For this review, take the finished solid that the model builds, in its own axes (mm). Face numbers are marked on the shaded views. A direction names the side the tool comes from. Give positions to 0.01 mm unless a question says otherwise; leave off trailing zeros. Loops run counter-clockwise (first coordinate to the right, second up) from the corner with the lowest first, then second, coordinate; pieces in that order, holes last.
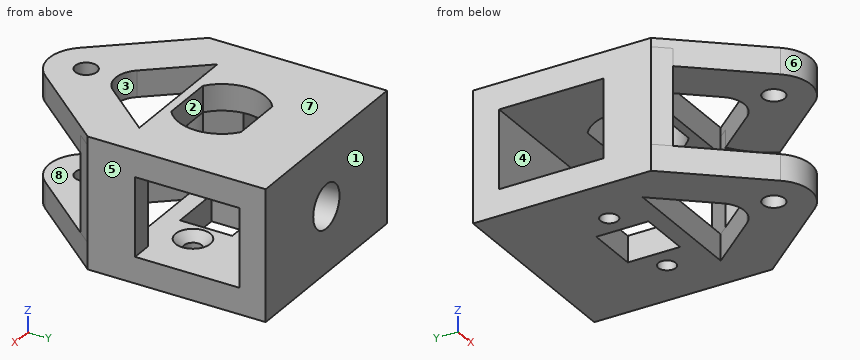
```python
from build123d import *

# Parameters (mm, degrees)
SKETCH1_R           = 1.25
BOSS_EXTRUDE1_DEPTH = 3
BOSS_EXTRUDE2_DEPTH = 14
FILLET1_R           = 1
FILLET3_R           = 3
CUT_EXTRUDE1_DEPTH  = 15
SKETCH8_W           = 23.078375234
SKETCH8_H           = 15
BOSS_EXTRUDE6_DEPTH = 15
SKETCH9_W           = 9
SKETCH9_H           = 12
CUT_EXTRUDE4_DEPTH  = 12.5
SKETCH10_W          = 3
SKETCH10_H          = 2
BOSS_EXTRUDE8_DEPTH = 11.5
CUT_EXTRUDE5_START  = 12
CUT_EXTRUDE5_DEPTH  = 3
SKETCH12_R          = 1
SKETCH12_W          = 6
SKETCH12_H          = 6
CUT_EXTRUDE6_DEPTH  = 3
CUT_EXTRUDE7_START  = 27.589042
SKETCH13_R          = 2.5
CUT_EXTRUDE7_DEPTH  = 4
CHAMFER1_SIZE       = 1


with BuildPart() as part:
    # Sketch1 → Boss-Extrude1 (new body)
    with BuildSketch(Plane.XY):
        with BuildLine():
            Line((-16.111441077, 12.589041521), (-3.255688883, -2.731847341))
            ThreePointArc((-3.255688883, -2.731847341), (0, -4.25), (3.255688883, -2.731847341))
            Line((3.255688883, -2.731847341), (16.111441077, 12.589041521))
            Line((16.111441077, 12.589041521), (9.111441077, 12.589041521))
            Line((9.111441077, 12.589041521), (0, 1.730448884))
            Line((0, 1.730448884), (-9.111441077, 12.589041521))
            Line((-9.111441077, 12.589041521), (-16.111441077, 12.589041521))
        make_face()
        Circle(SKETCH1_R, mode=Mode.SUBTRACT)
    boss_extrude1 = extrude(amount=BOSS_EXTRUDE1_DEPTH)

    # Sketch2 → Boss-Extrude2 (add)
    with BuildSketch(Plane.XY):
        with BuildLine():
            Line((16.111441077, 12.589041521), (9.111441077, 12.589041521))
            Line((9.111441077, 12.589041521), (6.505319132, 9.483186331))
            ThreePointArc((6.505319132, 9.483186331), (8.555448033, 7.684680147), (10.124424164, 5.453992606))
            Line((10.124424164, 5.453992606), (16.111441077, 12.589041521))
        make_face()
        with BuildLine():
            Line((-9.111441077, 12.589041521), (-16.111441077, 12.589041521))
            Line((-16.111441077, 12.589041521), (-10.124424164, 5.453992606))
            ThreePointArc((-10.124424164, 5.453992606), (-8.555448033, 7.684680147), (-6.505319132, 9.483186331))
            Line((-6.505319132, 9.483186331), (-9.111441077, 12.589041521))
        make_face()
    extrude(amount=BOSS_EXTRUDE2_DEPTH)

    # Mirror1: Boss-Extrude1 across plane
    add(boss_extrude1.mirror(Plane(origin=(0, 0, 7.5), x_dir=(1, 0, 0), z_dir=(0, 0, -1))))

    # Fillet1
    fillet1_edges = [part.edges().sort_by_distance(p)[0] for p in [
        (16.111441077, 12.589041521, 7.5),
        (-16.111441077, 12.589041521, 7.5),
    ]]
    fillet(fillet1_edges, radius=FILLET1_R)

    # Fillet3
    fillet3_edges = [part.edges().sort_by_distance(p)[0] for p in [
        (0, 1.730448884, 1.5),
        (0, 1.730448884, 13.5),
    ]]
    fillet(fillet3_edges, radius=FILLET3_R)

    # Sketch5 → Cut-Extrude1 (cut)
    with BuildSketch(Plane.XY):
        Polygon((11.539187617, 12.589041521), (11.539187617, 7.140042034), (16.111441077, 12.589041521), align=None)
        Polygon((-11.539187617, 12.589041521), (-11.539187617, 7.140042034), (-16.111441077, 12.589041521), align=None)
    extrude(amount=CUT_EXTRUDE1_DEPTH, mode=Mode.SUBTRACT)

    # Sketch8 → Boss-Extrude6 (add)
    with BuildSketch(Plane.XY):
        with Locations((0, 20.089041521)):
            Rectangle(SKETCH8_W, SKETCH8_H)
    extrude(amount=BOSS_EXTRUDE6_DEPTH)

    # Sketch9 → Cut-Extrude4 (cut, symmetric)
    with BuildSketch(Plane(origin=(0, 0, 0), x_dir=(0, 0, -1), z_dir=(1, 0, 0))):
        with Locations((-7.5, 18.589041521)):
            Rectangle(SKETCH9_W, SKETCH9_H)
    extrude(amount=CUT_EXTRUDE4_DEPTH, both=True, mode=Mode.SUBTRACT)

    # Sketch10 → Boss-Extrude8 (add, symmetric)
    with BuildSketch(Plane(origin=(0, 0, 0), x_dir=(0, 0, -1), z_dir=(1, 0, 0))):
        with Locations((-13.5, 11.589041521)):
            Rectangle(SKETCH10_W, SKETCH10_H)
        with Locations((-1.5, 11.589041521)):
            Rectangle(SKETCH10_W, SKETCH10_H)
    extrude(amount=BOSS_EXTRUDE8_DEPTH, both=True)

    # Sketch11 → Cut-Extrude5 (cut)
    with BuildSketch(Plane.XY.offset(CUT_EXTRUDE5_START)):
        with BuildLine():
            Line((-3, 11.589041521), (3, 11.589041521))
            ThreePointArc((3, 11.589041521), (5, 15.589041521), (3, 19.589041521))
            Line((3, 19.589041521), (-3, 19.589041521))
            ThreePointArc((-3, 19.589041521), (-5, 15.589041521), (-3, 11.589041521))
        make_face()
    extrude(amount=CUT_EXTRUDE5_DEPTH, mode=Mode.SUBTRACT)

    # Sketch12 → Cut-Extrude6 (cut)
    with BuildSketch(Plane.XY):
        with Locations((5.5, 15.589041521)):
            Circle(SKETCH12_R)
        with Locations((-5.5, 15.589041521)):
            Circle(SKETCH12_R)
        with Locations((0, 15.589041521)):
            Rectangle(SKETCH12_W, SKETCH12_H)
    extrude(amount=CUT_EXTRUDE6_DEPTH, mode=Mode.SUBTRACT)

    # Sketch13 → Cut-Extrude7 (cut)
    with BuildSketch(Plane(origin=(0, 0, 0), x_dir=(1, 0, 0), z_dir=(0, 1, 0)).offset(CUT_EXTRUDE7_START)):
        with Locations((0, -7.5)):
            Circle(SKETCH13_R)
    extrude(amount=-CUT_EXTRUDE7_DEPTH, mode=Mode.SUBTRACT)

    # Chamfer1
    chamfer1_edges = [part.edges().sort_by_distance(p)[0] for p in [
        (-6.5, 15.589041521, 3),
        (4.5, 15.589041521, 3),
    ]]
    chamfer(chamfer1_edges, length=CHAMFER1_SIZE)


solid = part.part
```
Item 1: Clearance check with flat-ended pins moving along their axes: pin 1 Ø0.9 at (x, z) = (3, 13.5) entering from -Y; pin 2 Ø1.5 at (x, z) = (-0.5, 1.5) entering from -Y; pin 3 Ø1.6 at (x, y) = (-5.5, 15.59) entering from -Z. State where each tip first meets the part, or that it passes through.
Answer:
pin 1: stops at y = -3.4
pin 2: stops at y = -4.25
pin 3: stops at z = 12
Item 2: Tool access review of the marked faces 1, 2, 3, 4 and 5: name each direction out of +Z, -Z, +X, -X, +Y, -Y from which nothing blocks a thin tool from reaching the whole face with its end or side.
Answer:
face 1: +Z, -Z, +X, -X, +Y
face 2: +Z
face 3: +Z, -Z
face 4: +X, -X
face 5: +Z, -Z, +X, +Y, -Y
Item 3: Take a section at D-D on y = 2.5. Give the boundary of the cut face in (x, z), and give its area (3 significant figures).
Answer:
outline: (-7.65, 0) - (7.65, 0) - (7.65, 3) - (-7.65, 3) - close; (-7.65, 12) - (7.65, 12) - (7.65, 15) - (-7.65, 15) - close
area: 91.7 mm2
Item 4: Take a section at B-B on y = 19. Give the boundary of the cut face in (x, z).
Answer:
outline: (-11.54, 0) - (11.54, 0) - (11.54, 3) - (-11.54, 3) - close; (-11.54, 12) - (-3.66, 12) - (-3.66, 15) - (-11.54, 15) - close; (3.66, 12) - (11.54, 12) - (11.54, 15) - (3.66, 15) - close
Item 5: Take a section at C-C on x = 5.5. Give the boundary of the cut face in (y, z).
Answer:
outline: (-0.06, 0) - (8.29, 0) - (8.29, 3) - (-0.06, 3) - close; (-0.06, 12) - (8.29, 12) - (8.29, 15) - (-0.06, 15) - close; (10.59, 0) - (14.59, 0) - (14.59, 2) - (13.59, 3) - (10.59, 3) - close; (10.59, 12) - (24.59, 12) - (24.59, 3) - (17.59, 3) - (16.59, 2) - (16.59, 0) - (27.59, 0) - (27.59, 15) - (10.59, 15) - close
Item 6: Take a section at A-A on z = 11. Give the boundary of the cut face in (x, y).
Answer:
outline: (-11.54, 7.14) - (-10.12, 5.45) arc R11.5 cw to (-6.51, 9.48) - (-9.11, 12.59) - (-11.54, 12.59) - close; (-11.54, 24.59) - (11.54, 24.59) - (11.54, 27.59) - (-11.54, 27.59) - close; (6.51, 9.48) arc R11.5 cw to (10.12, 5.45) - (11.54, 7.14) - (11.54, 12.59) - (9.11, 12.59) - close
Item 7: The part is to be moulded in two halves that separate along Z. For the marked faces 6, 7 and 8, say which applies: released by +Z, released by -Z, zero draft, split by the parting line, or undercut.
Answer:
face 6: zero draft
face 7: released by +Z
face 8: undercut
Item 8: For L1, parallel to Y at x = 0, z = 1.85; L2, parallel to Y at x = 0, z = 12.9; L3, parallel to Z at x = 9.75, y = 15, list the stretches that pass through material, from the lowest coordinate up.
Answer:
L1: y = -4.25 to -1.25, 1.25 to 3.4, 10.59 to 12.59, 18.59 to 27.59
L2: y = -4.25 to -1.25, 1.25 to 3.4, 10.59 to 11.59, 19.59 to 27.59
L3: z = 0 to 3, 12 to 15
